from build123d import *

# Parameters (mm, degrees)
SKETCH_1_W          = 136
SKETCH_1_H          = 8
EXTRUDE_1_DEPTH     = 8
SKETCH_2_R          = 1.5
CUT_EXTRUDE_1_DEPTH = 10
CUT_EXTRUDE_START   = -136
SKETCH_2_2_R        = 1.5
CUT_EXTRUDE_2_DEPTH = 10
SKETCH_3_R          = 6
SKETCH_3_R_2        = 4
CUT_EXTRUDE_3_DEPTH = 137


with BuildPart() as part:
    # Sketch 1 → Extrude 1 (new body)
    with BuildSketch(Plane.XY):
        with Locations((68, -4)):
            Rectangle(SKETCH_1_W, SKETCH_1_H)
    extrude(amount=EXTRUDE_1_DEPTH)

    # Sketch 2 → Cut-Extrude 1 (cut)
    with BuildSketch(Plane.ZY):
        with Locations((4, -4)):
            Circle(SKETCH_2_R)
    extrude(amount=-CUT_EXTRUDE_1_DEPTH, mode=Mode.SUBTRACT)

    # Sketch 2_2 → Cut-Extrude 2 (cut)
    with BuildSketch(Plane.ZY.offset(CUT_EXTRUDE_START)):
        with Locations((4, -4)):
            Circle(SKETCH_2_2_R)
    extrude(amount=CUT_EXTRUDE_2_DEPTH, mode=Mode.SUBTRACT)

    # Sketch 3 → Cut-Extrude 3 (cut, through all)
    with BuildSketch(Plane(origin=(136, 0, 0), x_dir=(0, 0, -1), z_dir=(1, 0, 0))):
        with Locations((-4, -4)):
            Circle(SKETCH_3_R)
        with Locations((-4, -4)):
            Circle(SKETCH_3_R_2, mode=Mode.SUBTRACT)
    extrude(amount=-CUT_EXTRUDE_3_DEPTH, mode=Mode.SUBTRACT)


solid = part.part
CAD build for the part. Positions are in the model's coordinates, mm. A direction names the side the tool comes from. Give positions to 0.01 mm unless a question says otherwise; leave off trailing zeros. Loops run counter-clockwise (first coordinate to the right, second up) from the corner with the lowest first, then second, coordinate; pieces in that order, holes last. Notation, with made-up numbers: M 89.5,-3.75 L 138.5,-3.75 A16 cw 138.5,19.25 Z; hole C -37,60.25 d4. An arc over 180 degrees is marked long. Answer in a Markdown table with one row per item. Add a question column.
Item 1: Band-saw the part on A-A on y = -4. Give the cut face in (x, z), then the cut area to 3 significant figures.
Item 2: Tool access for faces 1 (the face through (4.93, -3.55, 5.43)), 2 (the face through (126, -4, 4)), 3 (the face through (0, -2, 4)): list every direction of +Z, -Z, +X, -X, +Y, -Y with a clear straight run to the whole face (end or side of a thin tool).
Item 3: Band-saw the part on C-C on x = 75. Give the cut face in (y, z), then the cut area to 3 significant figures.
Item 4: Probe probe 1 along Y at (x, z) = (4.5, 4); probe 2 along X at (y, z) = (-5, 5); probe 3 along Z at (x, y) = (72.5, -2.75). List the from-to ranges inside material, lowest first.
Item 5: Band-saw the part on B-B on z = 4. Give the cut face in (x, y).
Item 6: Mould opens along Y. For faces 4 (the face through (10, -4, 4)), 5 (the face through (131.07, -3.55, 5.43)), 6 (the face through (68.952, -7.905, 4.867)), 7 (the face through (136, -2, 4)) say: +Y half, -Y half, draft (parallel to the pull), parting line (faces both ways), or undercut.
Item 7: Drop flat-ended pins along their axis: P1, Ø2.5, axis at y = -4, z = 4, coming from the +X side; P2, Ø3, axis at x = 55, y = -6.5, coming from the -Z side; P3, Ø2, axis at x = 118, z = 2, coming from the +Y side. Give the stop position or say it passes through.
Reply:
| question | item | result |
|---|---|---|
| 1 | outline | M 0,0 L 136,0 L 136,2.5 L 126,2.5 L 126,5.5 L 136,5.5 L 136,8 L 0,8 L 0,5.5 L 10,5.5 L 10,2.5 L 0,2.5 Z |
| 1 | area | 1,030 mm^2 |
| 2 | face 1 | -X |
| 2 | face 2 | +X |
| 2 | face 3 | +Z, -Z, -X, +Y, -Y |
| 3 | outline | C -4,4 d8 |
| 3 | area | 50.3 mm^2 |
| 4 | probe 1 | y = -8 to -5.5, -2.5 to 0 |
| 4 | probe 2 | x = 10 to 126 |
| 4 | probe 3 | z = 0.2 to 7.8 |
| 5 | outline | M 0,-8 L 136,-8 L 136,-5.5 L 126,-5.5 L 126,-2.5 L 136,-2.5 L 136,0 L 0,0 L 0,-2.5 L 10,-2.5 L 10,-5.5 L 0,-5.5 Z |
| 6 | face 4 | undercut |
| 6 | face 5 | undercut |
| 6 | face 6 | parting line |
| 6 | face 7 | draft |
| 7 | P1 | stops at x = 126 |
| 7 | P2 | stops at z = 0.13 |
| 7 | P3 | stops at y = -0.13 |
